Geometry: see drawing. Coordinates: mm, zero at the bounding-box minimum. Coordinates: 2 decimals unless noted, no trailing zeros. Order: outer loops, then holes, each group sorted by start corner. A loop starts at its lowest first (then second) coordinate and runs counter-clockwise, first axis right, second up. Notation, with made-up numbers: (71, 14.5) - (99, 14.5) arc R35 ccw to (99, 51.5) - close; hole circle Ø1 at (80.5, -6). An arc over 180 degrees is marked (long way). Use a Markdown table: item, result. Add a question column.
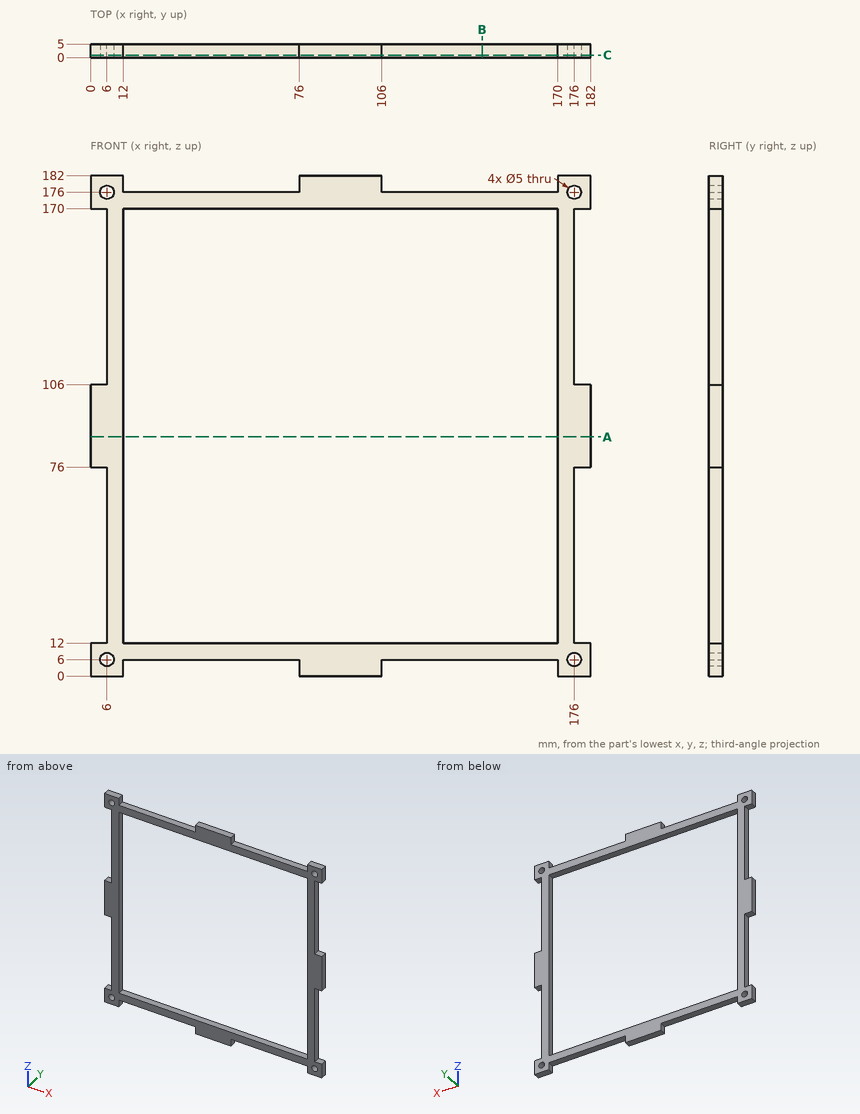
1) Section query C-C (y = 0.95). Give the number of separate pieces and of enclosed holes in the cut face, and give its area (3 significant figures).
2) First-contact query: pin 1 (2.5 mm diameter, centred on x = 45, y = 3, fed in from -Z); pin 2 (3 mm diameter, centred on x = 150, y = 3, fed in from +Z); pin 3 (6.5 mm diameter, centred on x = 6, z = 176, fed in from -Y); pin 4 (2.5 mm diameter, centred on y = 2, z = 51, fed in from -X). Flat tips, straight axial feed; report the tip coordinate or a pass-through.
3) Section query A-A (z = 87). Return the cut outline in (x, y).
4) Line query: line 1 (X direction, y = 0.4, z = 46.5); line 2 (X direction, y = 0.95, z = 99). Output: solid intervals per line, ascending. Write a range as from..to.
5) Section query B-B (x = 142.5). Return the cut outline in (y, z).
From the geometry:
| question | item | result |
|---|---|---|
| 1 | separate pieces | 1 |
| 1 | enclosed holes | 5 |
| 1 | area | 5,010 mm^2 |
| 2 | pin 1 | stops at z = 6 |
| 2 | pin 2 | stops at z = 176 |
| 2 | pin 3 | stops at y = 0 |
| 2 | pin 4 | stops at x = 6 |
| 3 | outline | (0, 0) - (12, 0) - (12, 5) - (0, 5) - close; (170, 0) - (182, 0) - (182, 5) - (170, 5) - close |
| 4 | line 1 | x = 6..12, 170..176 |
| 4 | line 2 | x = 0..12, 170..182 |
| 5 | outline | (0, 6) - (5, 6) - (5, 12) - (0, 12) - close; (0, 170) - (5, 170) - (5, 176) - (0, 176) - close |
